The model under review builds one solid part; all positions refer to its coordinate system, in mm. Face numbers are marked on the shaded views. A direction names the side the tool comes from. Round coordinates to 2 decimals unless told otherwise and drop trailing zeros. Loops run counter-clockwise (first coordinate to the right, second up) from the corner with the lowest first, then second, coordinate; pieces in that order, holes last. Notation, with made-up numbers: (-5, 23) -> (54, 23) arc R18 cw to (54, 35) -> close; hole circle Ø3 at (28, 18). An arc over 180 degrees is marked (long way). Use a Markdown table: item, result. Add a question column.
1) Consider section A-A on x = 0. Give the boundary of the cut face in (y, z), plus the area to 3 significant figures.
2) Mouldability with a two-part tool opening along Y and no side actions: class the marked faces 1, 2 and 3 as released by +Y, released by -Y, zero draft, split by the parting line, or undercut.
3) Insertion check: pin 1 (4 mm diameter, centred on y = -6.5, z = 24, fed in from +X); pin 2 (6 mm diameter, centred on y = -8.5, z = 6, fed in from -X); pin 3 (10.5 mm diameter, centred on x = 0, y = 0, fed in from -Z); pin 4 (4 mm diameter, centred on y = 6, z = 7.5, fed in from +X). Each pin has a flat end and moves straight along its axis. Give the tip position at first contact, or say it passes through.
4) For the marked faces 4 and 5, list the 3-axis set-ups (+Z, -Z, +X, -X, +Y, -Y) from which the entire face can be reached by the end or side of a thin tool; tool diameter is ignored.
5) Consider section C-C on z = 28.5. Give the boundary of the cut face in (x, y).
6) Consider section D-D on z = 4. Give the boundary of the cut face in (x, y), plus the area to 3 significant figures.
7) Wall thickness on probe 1 along X at (y, z) = (0, 12.5); probe 2 along Z at (x, y) = (0.75, 3.25): over which ranges is each line inside the solid? List them lowest first.
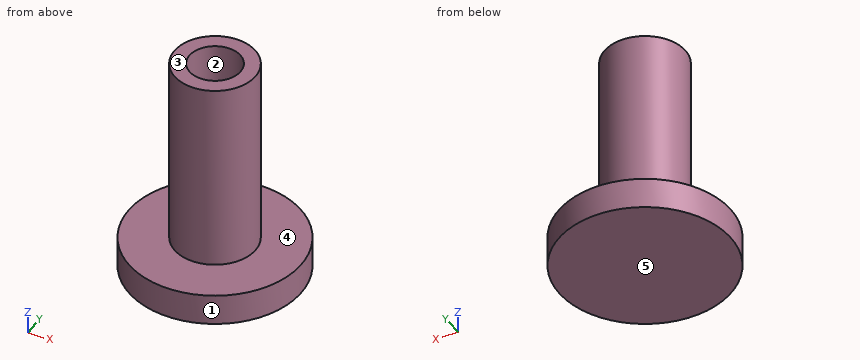
from build123d import *

# Parameters (mm, degrees)
F0_W   = 2.4
F0_H   = 30.767596
F0_W_2 = 4.1
F0_H_2 = 5
F0_W_3 = 7.320878


with BuildPart() as f1:
    # F0 (on Front) → F1 (revolve)
    with BuildSketch(Plane.XZ):
        with Locations((5.3, 20.383798)):
            Rectangle(F0_W, F0_H)
    revolve(axis=Axis((0, 0, 17.953249), (0, 0, -1)))

    # F0 (on Front) → F2 (revolve)
    with BuildSketch(Plane.XZ):
        with Locations((2.05, 2.5)):
            Rectangle(F0_W_2, F0_H_2)
        with Locations((5.3, 2.5)):
            Rectangle(F0_W, F0_H_2)
        with Locations((10.160439, 2.5)):
            Rectangle(F0_W_3, F0_H_2)
    revolve(axis=Axis((0, 0, 2.5), (0, 0, -1)))


solid = f1.part
Result set:
| question | item | result |
|---|---|---|
| 1 | outline | (-13.82, 0) -> (13.82, 0) -> (13.82, 5) -> (6.5, 5) -> (6.5, 35.77) -> (4.1, 35.77) -> (4.1, 5) -> (-4.1, 5) -> (-4.1, 35.77) -> (-6.5, 35.77) -> (-6.5, 5) -> (-13.82, 5) -> close |
| 1 | area | 286 mm2 |
| 2 | face 1 | split by the parting line |
| 2 | face 2 | undercut |
| 2 | face 3 | zero draft |
| 3 | pin 1 | x = 4.69 |
| 3 | pin 2 | x = -12.6 |
| 3 | pin 3 | z = 0 |
| 3 | pin 4 | x = 5.12 |
| 4 | face 4 | +Z |
| 4 | face 5 | -Z, +X, -X, +Y, -Y |
| 5 | outline | circle Ø13 at (0, 0); hole circle Ø8.2 at (0, 0) |
| 6 | outline | circle Ø27.64 at (0, 0) |
| 6 | area | 600 mm2 |
| 7 | probe 1 | -6.5 to -4.1, 4.1 to 6.5 |
| 7 | probe 2 | 0 to 5 |
